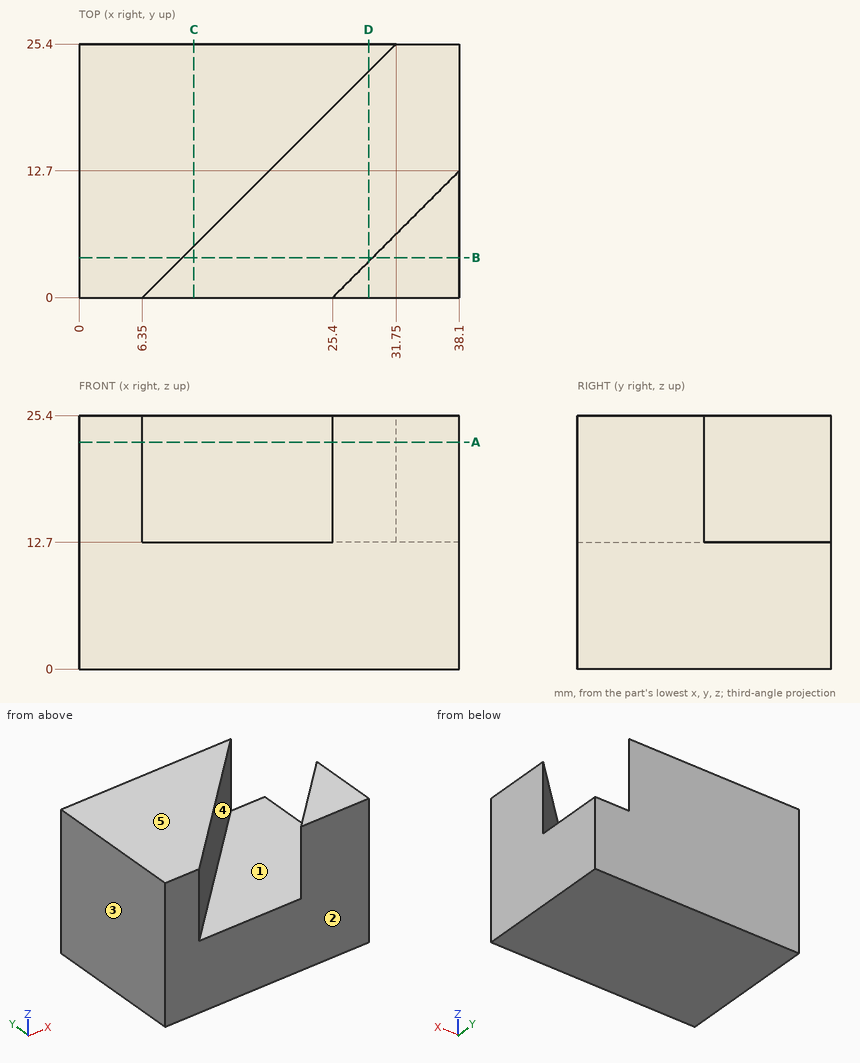
Here's the drawing with two shaded views (mm, measured from the low corner). I have some questions. A direction names the side the tool comes from. Round coordinates to 2 decimals unless told otherwise and drop trailing zeros. Loops run counter-clockwise (first coordinate to the right, second up) from the corner with the lowest first, then second, coordinate; pieces in that order, holes last.
Item 1: Suppose I cut it at A-A, the plane z = 22.75. Write out the boundary of the cut face in (x, y).
Item 2: Which directions (+Z, -Z, +X, -X, +Y, -Y) give clear straight access to the entire face, cutting with the end or side of a thin tool? Please do the marked faces 4 and 5.
Item 3: Will these pins go through, and if not, where does the flat tip stop? pin 1 Ø7.5 at (x, y) = (17, 8.5) entering from +Z; pin 2 Ø2 at (x, y) = (21.5, 6) entering from +Z.
Item 4: Suppose I cut it at B-B, the plane y = 4. Write out the boundary of the cut face in (x, z).
Item 5: If we mould it in two halves opening along Y, with no side actions, what happens to the marked faces 1, 2 and 3? For each: +Y half, -Y half, draft (parallel to the pull), parting line (faces both ways), or undercut.
Item 6: Suppose I cut it at C-C, the plane x = 11.5. Write out the boundary of the cut face in (y, z).
Item 7: Suppose I cut it at D-D, the plane x = 29. Write out the boundary of the cut face in (y, z).
Item 8: Please list where these lines run through material, in increasing order: L1, parallel to Z at x = 33.5, y = 16.75; L2, parallel to X at y = 11.75, z = 22; L3, parallel to X at y = 3.5, z = 21.5.
Reported:
1. outline: (0, 0) - (6.35, 0) - (31.75, 25.4) - (0, 25.4) - close; (25.4, 0) - (38.1, 0) - (38.1, 12.7) - close
2. face 4: +Z
2. face 5: +Z, +X, -X, +Y, -Y
3. pin 1: stops at z = 25.4
3. pin 2: stops at z = 12.7
4. outline: (0, 0) - (38.1, 0) - (38.1, 25.4) - (29.4, 25.4) - (29.4, 12.7) - (10.35, 12.7) - (10.35, 25.4) - (0, 25.4) - close
5. face 1: undercut
5. face 2: -Y half
5. face 3: draft
6. outline: (0, 0) - (25.4, 0) - (25.4, 25.4) - (5.15, 25.4) - (5.15, 12.7) - (0, 12.7) - close
7. outline: (0, 0) - (25.4, 0) - (25.4, 25.4) - (22.65, 25.4) - (22.65, 12.7) - (3.6, 12.7) - (3.6, 25.4) - (0, 25.4) - close
8. L1: z = 0 to 12.7
8. L2: x = 0 to 18.1, 37.15 to 38.1
8. L3: x = 0 to 9.85, 28.9 to 38.1
